Work out the finished part from the listing and answer in its coordinate system (mm). Face numbers are marked on the shaded views. A direction names the side the tool comes from. Give positions to 0.01 mm unless a question says otherwise; leave off trailing zeros. Order: outer loops, then holes, each group sorted by start corner. A loop starts at its lowest first (then second) coordinate and runs counter-clockwise, first axis right, second up. Notation, with made-up numbers: (-0.75, 59.5) - (54.25, 59.5) arc R9 ccw to (54.25, 73.5) - close; hole circle Ø1 at (81, -16). An arc over 180 degrees is marked (long way). Write each question's results on one line, items separated by ' | '.
Autodesk Inventor part; units mm, degrees
ref_plane "YZ Plane" through (0, 0, 0) normal (1, 0, 0) x (0, 1, 0)
ref_plane "XZ Plane" through (0, 0, 0) normal (0, 1, 0) x (-1, 0, 0)
ref_plane "XY Plane" through (0, 0, 0) normal (0, 0, 1) x (1, 0, 0)
sketch "Sketch1" plane through (0, 0, 0) normal (0, 1, 0) x (-1, 0, 0)
  line L0 (-3, -8) -> (3, -8)
  line L1 (3, -8) -> (3, 8)
  line L2 (3, 8) -> (-3, 8)
  line L3 (-3, 8) -> (-3, -8)
  line L4 (-3, -8) -> (3, 8) construction
  line L5 (3, -8) -> (-3, 8) construction
  point P0 (0, 0)
  dimension "d0" = 16
  dimension "d1" = 6
extrude "Extrusion1" add sketch "Sketch1" along normal blind 2.5
sketch "Sketch2" plane through (0, 2.5, 0) normal (0, 1, 0) x (1, 0, 0)
  line L0 (0, 5) -> (0, 2) construction
  line L1 (-1.25, 5) -> (-1.25, 2)
  line L2 (1.25, 2) -> (1.25, 5)
  arc A0 (1.25, 5) -> (-1.25, 5) centre (0, 5) ccw
  arc A1 (-1.25, 2) -> (1.25, 2) centre (0, 2) ccw
  line L3 (-3, -8) -> (3, -8)
  line L4 (-3, 8) -> (-3, -8)
  line L5 (-3, -8) -> (3, -8)
  line L6 (3, -8) -> (3, 8)
  line L7 (3, 8) -> (-3, 8)
  point P0 (0, 3.5)
  point P1 (0, 3.5)
  dimension "d4" = 2.5
  dimension "d7" = 6
  dimension "d8" = 3
  dimension "d9" = 3
  dimension "d28" = 3
extrude "Extrusion2" cut sketch "Sketch2" against normal through all contours A0 L2 A1 L1
sketch "Sketch3" plane through (3, 0, 8) normal (1, 0, 0) x (0, 0, -1)
  line L0 (16, 0) -> (0, 0)
  line L1 (16, 0) -> (2, 0)
  line L2 (2, 0) -> (2, 1)
  line L3 (2, 1) -> (16, 1)
  line L4 (16, 1) -> (16, 0)
  line L5 (0, 0) -> (0, 2.5)
  line L6 (0, 2.5) -> (16, 2.5)
  point P0 (8, 0)
  point P1 (2, 0)
  dimension "d12" = 2
  dimension "d13" = 1.5
extrude "Extrusion3" cut sketch "Sketch3" against normal through all
sketch "Sketch4" plane through (0, 2.5, 0) normal (0, 1, 0) x (1, 0, 0)
  line L0 (-3, 8) -> (-3, -8)
  line L1 (3, -8) -> (3, 8)
  arc A0 (-3, -6) -> (3, -6) centre (0, -4.75) ccw
  line L2 (-3, -8) -> (3, -8)
  point P0 (0, 0)
  point P1 (-2, 6)
  point P2 (2, 6)
  point P3 (3, 8)
  point P4 (0, -8)
  point P5 (-2.2361, -8)
  dimension "d17" = 2
extrude "Extrusion4" cut sketch "Sketch4" against normal through all
sketch "Sketch5" plane through (0, 2.5, 0) normal (0, 1, 0) x (1, 0, 0)
  line L0 (3, -6) -> (3, 8)
  line L1 (3, 8) -> (-3, 8)
  line L2 (-3, 8) -> (-3, -6)
  arc A0 (1.25, 5) -> (-1.25, 5) centre (0, 5) ccw
  arc A1 (3, 4) -> (0, 7.5) centre (-1.8689, 2.8624) ccw
  arc A2 (0, 7.5) -> (-3, 4) centre (1.8689, 2.8624) ccw
  point P0 (0, 0)
  point P1 (-3, 6.2041)
  point P2 (0, 6.25)
  point P3 (0, 6.25)
  dimension "d23" = 5
  dimension "d24" = 4
  dimension "d25" = 0.5
extrude "Extrusion5" cut sketch "Sketch5" against normal through all
sketch "Sketch6" plane through (-3, 1, 6) normal (0, -1, 0) x (1, 0, 0)
  line L0 (6.1469, -11) -> (-0.0299, -11)
  line L1 (-0.0299, -11) -> (-0.0299, -13.5)
  line L2 (-0.0299, -13.5) -> (6.1469, -13.5)
  line L3 (6.1469, -13.5) -> (6.1469, -11)
  arc A0 (1.75, -11) -> (4.25, -11) centre (3, -11) ccw
  point P0 (3, -6)
  point P1 (3, -13.5)
  point P2 (1.75, -11)
extrude "Extrusion6" cut sketch "Sketch6" against normal blind 0.3 contours L3 L2 L1 L0 A0
sketch "Sketch7" plane through (0, 2.5, 0) normal (0, 1, 0) x (1, 0, 0)
  line L0 (3, -6) -> (3, 4)
  line L1 (-3, 4) -> (-3, -6)
  line L2 (-3, -4.25) -> (3, -4.25)
  arc A0 (-1.25, 2) -> (1.25, 2) centre (0, 2) ccw
  arc A1 (-3, -6) -> (3, -6) centre (0, -4.75) ccw
  point P0 (0, 0)
  point P1 (0, 0.75)
  dimension "d29" = 5
extrude "Extrusion7" cut sketch "Sketch7" against normal through all
fillet "Fillet2" radius 2 2 edges at (3, 1.75, 4.25) (-3, 1.75, 4.25)
properties part number "Carrier Tab V2"
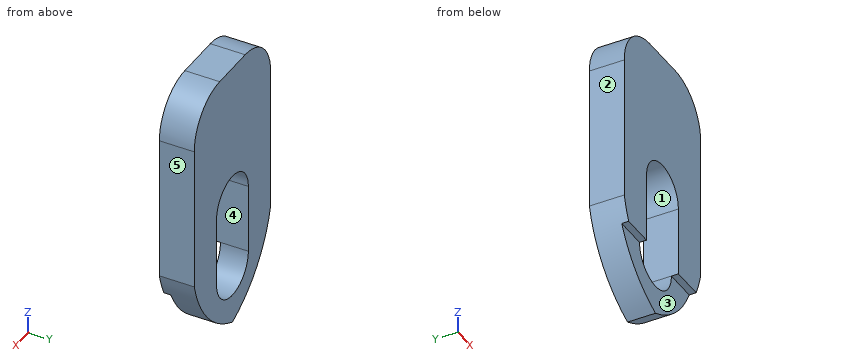
1. A cutting plane is placed at A-A, the plane z = -2.5. Write down the section's boundary in (x, y).
Answer list:
outline: (-3, 1) - (-1.25, 1) - (-1.25, 2.5) - (-3, 2.5) - close; (1.25, 1) - (3, 1) - (3, 2.5) - (1.25, 2.5) - close
2. A tool of negligible diameter and unlimited length cuts with its end or side. For the marked faces 4 and 5, from which of +Z, -Z, +X, -X, +Y, -Y can it reach the whole face along a straight path? Write none if from no direction.
Answer list:
face 4: +Y, -Y | face 5: +Z, -Z, +X, +Y, -Y
3. Given P1, Ø1, axis at x = 0, z = -2, coming from the +Y side, flat-ended and moving along its own axis, determine where the tip first touches the part or whether it passes through.
Answer list:
P1: through
4. A cutting plane is placed at B-B, the plane y = 1.65. Write down the section's boundary in (x, z), then the cut area to 3 significant figures.
Answer list:
outline: (-3, -4) arc R5 ccw to (0, -7.5) arc R5 ccw to (3, -4) - (3, 2.25) arc R2 ccw to (1, 4.25) - (-1, 4.25) arc R2 ccw to (-3, 2.25) - close; hole (-1.25, -5) arc R1.25 ccw to (1.25, -5) - (1.25, -2) arc R1.25 ccw to (-1.25, -2) - close | area: 49.4 mm^2
5. A cutting plane is placed at D-D, the plane z = 3.5. Write down the section's boundary in (x, y).
Answer list:
outline: (-2.56, 1) - (2.56, 1) - (2.56, 2.5) - (-2.56, 2.5) - close
6. Determine the mould class of the marked faces 1, 2 and 3 for opening direction X: +X half, -X half, draft (parallel to the pull), parting line (faces both ways), or undercut.
Answer list:
face 1: undercut | face 2: -X half | face 3: draft
7. Straight lines are drawn through the part: line 1 (X direction, y = 1.9, z = -3); line 2 (Z direction, x = 0, y = 1.2); line 3 (X direction, y = 1.55, z = -5.5). For each, find the intervals that lie inside material, in ascending order. Write a range as [from, to].
Answer list:
line 1: [-3, -1.25], [1.25, 3] | line 2: [-0.75, 4.25] | line 3: [-2.38, -1.15], [1.15, 2.38]
8. A cutting plane is placed at C-C, the plane x = -2.25. Write down the section's boundary in (y, z), then the cut area to 3 significant figures.
Answer list:
outline: (1, -5) - (1.3, -5) - (1.3, -5.7) - (2.5, -5.7) - (2.5, 3.81) - (1, 3.81) - close | area: 14.1 mm^2
